from build123d import *

# Parameters (mm, degrees)
BOSS_EXTRUDE1_DEPTH = 2.5
SKETCH4_R           = 1.78
CUT_EXTRUDE1_DEPTH  = 1.5
FILLET1_R           = 1.5


with BuildPart() as part:
    # Sketch2 → Boss-Extrude1 (new body)
    with BuildSketch(Plane(origin=(0, 0, 0), x_dir=(1, 0, 0), z_dir=(0, 1, 0))):
        Polygon((-21.216153836, 11.741903429), (-21.216153836, 8.241903429), (-3.016153836, -0.958096571), (4.783846164, -0.958096571), (12.783846164, 3.741903429), (12.783846164, 11.741903429), align=None)
    extrude(amount=BOSS_EXTRUDE1_DEPTH)

    # Sketch4 → Cut-Extrude1 (cut)
    with BuildSketch(Plane(origin=(0, 2.5, 0), x_dir=(1, 0, 0), z_dir=(0, 1, 0))):
        with Locations((-17.966153836, 8.241903429)):
            Circle(SKETCH4_R)
        with Locations(Location((9.533846164, 8.241903429, 0), (0, 0, 90))):
            Circle(SKETCH4_R)
    extrude(amount=-CUT_EXTRUDE1_DEPTH, mode=Mode.SUBTRACT)

    # Fillet1
    # the kernel refuses this fillet: 1.5 mm, written as the material it takes off along each edge
    with BuildSketch(Plane(origin=(4.375823919, 1.5, -0.541903429), x_dir=(0.5065490486308655, 0, 0.8622111466057285), z_dir=(0, -1, 0))) as fillet1_piece_1_section:
        Polygon((0, 0), (FILLET1_R, 0), (FILLET1_R, FILLET1_R * 0.272014830087), (FILLET1_R * 0.862211146606, FILLET1_R * 0.506549048631), align=None)
    fillet1_piece_1 = extrude(amount=FILLET1_R, mode=Mode.PRIVATE)
    fillet1_piece_1 = fillet1_piece_1 - Plane(origin=(4.375823919, 1.5, -0.541903429), x_dir=(-0.2624774784569825, 0, -0.964938118898235), z_dir=(0, -1, 0)) * Sphere(FILLET1_R, mode=Mode.PRIVATE)
    add(fillet1_piece_1, mode=Mode.SUBTRACT)
    with BuildSketch(Plane(origin=(-2.658577298, 1.5, -0.541903429), x_dir=(-0.4511321826525704, 0, 0.8924571439431296), z_dir=(0, -1, 0))) as fillet1_piece_2_section:
        Polygon((0, 0), (FILLET1_R, 0), (FILLET1_R, -FILLET1_R * 0.238384358714), (FILLET1_R * 0.892457143943, -FILLET1_R * 0.451132182653), align=None)
    fillet1_piece_2 = extrude(amount=FILLET1_R, mode=Mode.PRIVATE)
    fillet1_piece_2 = fillet1_piece_2 - Plane(origin=(-2.658577298, 1.5, -0.541903429), x_dir=(0.23188667065710186, 0, -0.972742808748317), z_dir=(0, -1, 0)) * Sphere(FILLET1_R, mode=Mode.PRIVATE)
    add(fillet1_piece_2, mode=Mode.SUBTRACT)
    with BuildSketch(Plane(origin=(-19.716153836, 1.5, -10.241903429), x_dir=(0, -1, 0), z_dir=(-1, 0, 0))) as fillet1_piece_3_section:
        Polygon((0, 0), (FILLET1_R, 0), (FILLET1_R, -FILLET1_R), (0, -FILLET1_R), align=None)
    fillet1_piece_3 = extrude(amount=FILLET1_R, mode=Mode.PRIVATE)
    fillet1_piece_3 = fillet1_piece_3 - Plane(origin=(-19.716153836, 1.5, -10.241903429), x_dir=(0, 0.7071067811865475, 0.7071067811865475), z_dir=(-1, 0, 0)) * Sphere(FILLET1_R, mode=Mode.PRIVATE)
    add(fillet1_piece_3, mode=Mode.SUBTRACT)
    with BuildSketch(Plane(origin=(-19.716153836, 1.5, -9.164414646), x_dir=(-0.4511321826525704, 0, 0.8924571439431296), z_dir=(0, -1, 0))) as fillet1_piece_4_section:
        Polygon((0, 0), (FILLET1_R, 0), (FILLET1_R, FILLET1_R * 0.615007478031), (FILLET1_R * 0.451132182653, FILLET1_R * 0.892457143943), align=None)
    fillet1_piece_4 = extrude(amount=FILLET1_R, mode=Mode.PRIVATE)
    fillet1_piece_4 = fillet1_piece_4 - Plane(origin=(-19.716153836, 1.5, -9.164414646), x_dir=(0.8518016737047921, 0, -0.5238643991279756), z_dir=(0, -1, 0)) * Sphere(FILLET1_R, mode=Mode.PRIVATE)
    add(fillet1_piece_4, mode=Mode.SUBTRACT)
    with BuildSketch(Plane(origin=(11.283846164, 1.5, -4.600366498), x_dir=(1, 0, 0), z_dir=(0, -1, 0))) as fillet1_piece_5_section:
        Polygon((0, 0), (FILLET1_R, 0), (FILLET1_R, FILLET1_R * 0.572308712676), (FILLET1_R * 0.506549048631, FILLET1_R * 0.862211146606), align=None)
    fillet1_piece_5 = extrude(amount=FILLET1_R, mode=Mode.PRIVATE)
    fillet1_piece_5 = fillet1_piece_5 - Plane(origin=(11.283846164, 1.5, -4.600366498), x_dir=(-0.8679138922240112, 0, -0.49671468237265487), z_dir=(0, -1, 0)) * Sphere(FILLET1_R, mode=Mode.PRIVATE)
    add(fillet1_piece_5, mode=Mode.SUBTRACT)
    with BuildSketch(Plane(origin=(11.283846164, 1.5, -10.241903429), x_dir=(0, 0, -1), z_dir=(0, -1, 0))) as fillet1_piece_6_section:
        Polygon((0, 0), (FILLET1_R, 0), (FILLET1_R, FILLET1_R), (0, FILLET1_R), align=None)
    fillet1_piece_6 = extrude(amount=FILLET1_R, mode=Mode.PRIVATE)
    fillet1_piece_6 = fillet1_piece_6 - Plane(origin=(11.283846164, 1.5, -10.241903429), x_dir=(-0.7071067811865477, 0, 0.7071067811865474), z_dir=(0, -1, 0)) * Sphere(FILLET1_R, mode=Mode.PRIVATE)
    add(fillet1_piece_6, mode=Mode.SUBTRACT)
    with BuildSketch(Plane(origin=(4.783846164, 1.5, 0.958096571), x_dir=(0.8622111466057288, 0, -0.506549048630865), z_dir=(0, 1, 0))) as fillet1_piece_7:
        with BuildLine():
            CenterArc((FILLET1_R * 0.272014830087, FILLET1_R), FILLET1_R, 239.565764247, 30.434235753)
            Line((-FILLET1_R * 0.234534218543, FILLET1_R * 0.137788853394), (0, 0))
            Line((0, 0), (FILLET1_R * 0.272014830087, 0))
        make_face()
    extrude(amount=2.020055613, mode=Mode.SUBTRACT)
    with BuildSketch(Plane(origin=(-3.016153836, 1.5, 0.958096571), x_dir=(1, 0, 0), z_dir=(0, 1, 0))) as fillet1_piece_8:
        with BuildLine():
            CenterArc((FILLET1_R * 0.238384358714, FILLET1_R), FILLET1_R, 243.183653156, 26.816346844)
            Line((-FILLET1_R * 0.212747823939, FILLET1_R * 0.107542856057), (0, 0))
            Line((0, 0), (FILLET1_R * 0.238384358714, 0))
        make_face()
    extrude(amount=1.893941345, mode=Mode.SUBTRACT)
    with BuildSketch(Plane(origin=(-21.216153836, 0, -10.241903429), x_dir=(0, 1, 0), z_dir=(0, 0, 1))) as fillet1_piece_9:
        with BuildLine():
            CenterArc((FILLET1_R, -FILLET1_R), FILLET1_R, 90, 90)
            Line((0, -FILLET1_R), (0, 0))
            Line((0, 0), (FILLET1_R, 0))
        make_face()
    extrude(amount=1.077488783, mode=Mode.SUBTRACT)
    with BuildSketch(Plane(origin=(-20.39285211, 0, -7.825728931), x_dir=(0.4511321826525704, 0, -0.8924571439431296), z_dir=(0.8924571439431296, 0, 0.4511321826525704))) as fillet1_piece_10:
        with BuildLine():
            CenterArc((FILLET1_R, FILLET1_R), FILLET1_R, 180, 90)
            Line((0, FILLET1_R), (0, 0))
            Line((0, 0), (FILLET1_R, 0))
        make_face()
    extrude(amount=19.113048345, mode=Mode.SUBTRACT)
    with BuildSketch(Plane(origin=(-2.658577298, 0, 0.958096571), x_dir=(0, 1, 0), z_dir=(1, 0, 0))) as fillet1_piece_11:
        with BuildLine():
            CenterArc((FILLET1_R, -FILLET1_R), FILLET1_R, 90, 90)
            Line((0, -FILLET1_R), (0, 0))
            Line((0, 0), (FILLET1_R, 0))
        make_face()
    extrude(amount=7.034401217, mode=Mode.SUBTRACT)
    with BuildSketch(Plane(origin=(5.135647492, 0, 0.751413291), x_dir=(0, 1, 0), z_dir=(0.8622111466057285, 0, -0.5065490486308655))) as fillet1_piece_12:
        with BuildLine():
            CenterArc((FILLET1_R, -FILLET1_R), FILLET1_R, 90, 90)
            Line((0, -FILLET1_R), (0, 0))
            Line((0, 0), (FILLET1_R, 0))
        make_face()
    extrude(amount=8.011984387, mode=Mode.SUBTRACT)
    with BuildSketch(Plane(origin=(12.783846164, 1.5, -3.741903429), x_dir=(0, 0, -1), z_dir=(0, 1, 0))) as fillet1_piece_13:
        with BuildLine():
            CenterArc((FILLET1_R * 0.572308712676, FILLET1_R), FILLET1_R, 210.434235753, 59.565764247)
            Line((-FILLET1_R * 0.289902433929, FILLET1_R * 0.493450951369), (0, 0))
            Line((0, 0), (FILLET1_R * 0.572308712676, 0))
        make_face()
    extrude(amount=3.146157673, mode=Mode.SUBTRACT)
    with BuildSketch(Plane(origin=(12.783846164, 0, -4.600366498), x_dir=(0, 1, 0), z_dir=(0, 0, -1))) as fillet1_piece_14:
        with BuildLine():
            CenterArc((FILLET1_R, -FILLET1_R), FILLET1_R, 90, 90)
            Line((0, -FILLET1_R), (0, 0))
            Line((0, 0), (FILLET1_R, 0))
        make_face()
    extrude(amount=5.641536931, mode=Mode.SUBTRACT)
    with BuildSketch(Plane(origin=(11.283846164, 0, -11.741903429), x_dir=(0, 0, 1), z_dir=(-1, 0, 0))) as fillet1_piece_15:
        with BuildLine():
            CenterArc((FILLET1_R, FILLET1_R), FILLET1_R, 180, 90)
            Line((0, FILLET1_R), (0, 0))
            Line((0, 0), (FILLET1_R, 0))
        make_face()
    extrude(amount=31, mode=Mode.SUBTRACT)
    with BuildSketch(Plane(origin=(12.783846164, 1.5, -11.741903429), x_dir=(0, 0, 1), z_dir=(0, 1, 0))) as fillet1_piece_16:
        with BuildLine():
            CenterArc((FILLET1_R, -FILLET1_R), FILLET1_R, 90, 90)
            Line((0, -FILLET1_R), (0, 0))
            Line((0, 0), (FILLET1_R, 0))
        make_face()
    extrude(amount=4.75, mode=Mode.SUBTRACT)
    with BuildSketch(Plane(origin=(-21.216153836, 1.5, -8.241903429), x_dir=(0, 0, -1), z_dir=(0, 1, 0))) as fillet1_piece_17:
        with BuildLine():
            CenterArc((FILLET1_R * 0.615007478031, -FILLET1_R), FILLET1_R, 90, 63.183653156)
            Line((-FILLET1_R * 0.277449665912, -FILLET1_R * 0.548867817347), (0, 0))
            Line((0, 0), (FILLET1_R * 0.615007478031, 0))
        make_face()
    extrude(amount=3.306278043, mode=Mode.SUBTRACT)
    with BuildSketch(Plane(origin=(-21.216153836, 1.5, -11.741903429), x_dir=(0, 0, 1), z_dir=(0, 1, 0))) as fillet1_piece_18:
        with BuildLine():
            CenterArc((FILLET1_R, FILLET1_R), FILLET1_R, 180, 90)
            Line((0, FILLET1_R), (0, 0))
            Line((0, 0), (FILLET1_R, 0))
        make_face()
    extrude(amount=4.75, mode=Mode.SUBTRACT)


solid = part.part
Geometry check sheet. Reference: the model listing, model coordinates, mm. A direction names the side the tool comes from. Coordinates: 2 decimals unless noted, no trailing zeros. Order: outer loops, then holes, each group sorted by start corner. A loop starts at its lowest first (then second) coordinate and runs counter-clockwise, first axis right, second up. Notation, with made-up numbers: (-37, 37) -> (-29, 37) arc R22 cw to (-29, 61) -> close; hole circle Ø6 at (73.25, -18.5). An arc over 180 degrees is marked (long way). Use a Markdown table: item, result. Add a question column.
1. Cross-section at C-C (y = 0.4). Enter the section's corners in (x, z).
2. Cross-section at B-B (y = 1.9). Enter the section's corners in (x, z), and give its area (3 significant figures).
3. Cross-section at A-A (x = 2). Enter the section's corners in (y, z), and give its area (3 significant figures).
4. Mould release check, pull along X, two halves, no side actions. Record for faces 1 (the face through (-4, 2, -11.742)), 2 (the face through (-21, 1.99, -8.39)), 3 (the face through (10.216, 1.76, -9.886)): pulls with the +X half, pulls with the -X half, needs draft (parallel to the pull), parting line crosses it, or undercut.
5. Set-up check for faces 4 (the face through (-17.107, 1.76, -9.801)), 5 (the face through (12.4, 0.5, -7.4)): record each of +Z, -Z, +X, -X, +Y, -Y from which the full face is reachable in a straight line by a thin tool's end or side.
6. Material ranges on L1, parallel to X at y = 1.75, z = -8.25; L2, parallel to Y at x = 8.5, z = -7; L3, parallel to Z at x = 9.5, y = 1.85, recorded low to high.
7. Go/stop test with flat-tipped pins: pin 1 Ø1 at (y, z) = (1.5, -3) entering from +X; pin 2 Ø1.1 at (x, z) = (-18, -8.5) entering from +Y. Record where each tip stops, or that it passes through.
Filled sheet:
| question | item | result |
|---|---|---|
| 1 | outline | (-20.74, -10.24) arc R1.02 ccw to (-19.72, -11.26) -> (11.28, -11.26) arc R1.02 ccw to (12.3, -10.24) -> (12.3, -4.6) arc R1.02 ccw to (11.8, -3.72) -> (4.89, 0.34) arc R1.02 ccw to (4.38, 0.48) -> (-2.66, 0.48) arc R1.02 ccw to (-3.12, 0.37) -> (-20.18, -8.25) arc R1.02 ccw to (-20.74, -9.16) -> close |
| 2 | outline | (-21.22, -10.24) arc R1.5 ccw to (-19.72, -11.74) -> (11.28, -11.74) arc R1.5 ccw to (12.78, -10.24) -> (12.78, -4.6) arc R1.5 ccw to (12.04, -3.31) -> (5.14, 0.75) arc R1.5 ccw to (4.38, 0.96) -> (-2.66, 0.96) arc R1.5 ccw to (-3.34, 0.8) -> (-17.73, -6.48) arc R1.78 cw (long way) to (-19.53, -7.39) -> (-20.39, -7.83) arc R1.5 ccw to (-21.22, -9.16) -> close; hole circle Ø3.56 at (9.53, -8.24) |
| 2 | area | 309 mm2 |
| 3 | outline | (0, -10.24) arc R1.5 ccw to (1.5, -11.74) -> (2.5, -11.74) -> (2.5, 0.96) -> (1.5, 0.96) arc R1.5 ccw to (0, -0.54) -> close |
| 3 | area | 30.8 mm2 |
| 4 | face 1 | needs draft |
| 4 | face 2 | pulls with the -X half |
| 4 | face 3 | undercut |
| 5 | face 4 | +Y |
| 5 | face 5 | +Z, -Z, +X, -Y |
| 6 | L1 | -20.91 to -19.75, -16.19 to 7.75, 11.31 to 12.78 |
| 6 | L2 | 0 to 1 |
| 6 | L3 | -11.74 to -10.02, -6.46 to -1.81 |
| 7 | pin 1 | x = 12.3 |
| 7 | pin 2 | y = 1 |
